Geometry: final body of the model. Coordinates: model frame, mm. Give positions to 0.01 mm unless a question says otherwise; leave off trailing zeros. Write each loop counter-clockwise with the first axis right and the second up, starting at its lowest first coordinate (ties: lowest second). Pieces come first, ordered by that corner, then holes. Notation, with made-up numbers: (-12, 84) -> (7, 84) arc R17 ccw to (7, 112) -> close; hole circle Ø3 at (52.5, 32). An arc over 180 degrees is marked (long way). Answer as a JSON object with one key per item and string values.
from build123d import *

# Parameters (mm, degrees)
BOSS_EXTRUDE1_DEPTH      = 2.159
BOSS_EXTRUDE1_DEPTH_BACK = 2.159
SKETCH6_W                = 177.8
SKETCH6_H                = 279.4
SKETCH6_W_2              = 152.4
SKETCH6_H_2              = 254
BOSS_EXTRUDE2_DEPTH      = 8.89
SKETCH7_R                = 3
CUT_EXTRUDE2_DEPTH       = 251.170207847


with BuildPart() as part:
    # Sketch3 → Boss-Extrude1 (new, two sides: drawn at the far end of the back side and taken through both)
    with BuildSketch(Plane.XY.offset(-BOSS_EXTRUDE1_DEPTH_BACK)):
        Polygon((-149.987, 177.025), (-126.987, 200.025), (126.987, 200.025), (149.987, 177.025), (149.987, -177.025), (126.987, -200.025), (-126.987, -200.025), (-149.987, -177.025), align=None)
    extrude(amount=BOSS_EXTRUDE1_DEPTH + BOSS_EXTRUDE1_DEPTH_BACK)

    # Sketch6 → Boss-Extrude2 (add)
    with BuildSketch(Plane(origin=(0, 0, -2.159), x_dir=(-1, 0, 0), z_dir=(0, 0, -1))):
        Rectangle(SKETCH6_W, SKETCH6_H)
        Rectangle(SKETCH6_W_2, SKETCH6_H_2, mode=Mode.SUBTRACT)
    extrude(amount=-BOSS_EXTRUDE2_DEPTH)

    # Sketch7 → Cut-Extrude2 (cut, through all)
    with BuildSketch(Plane(origin=(0, 0, -2.159), x_dir=(-1, 0, 0), z_dir=(0, 0, -1))):
        with Locations((133.477, 178.943)):
            Circle(SKETCH7_R)
        with Locations((-133.477, 178.943)):
            Circle(SKETCH7_R)
        with Locations((-133.477, -178.943)):
            Circle(SKETCH7_R)
        with Locations((133.477, -178.943)):
            Circle(SKETCH7_R)
    extrude(amount=-CUT_EXTRUDE2_DEPTH, mode=Mode.SUBTRACT)


solid = part.part
Q1. Cut plane B-B (y = -116). Return the cut outline in (x, z).
Values:
{"outline": "(-149.99, -2.16) -> (149.99, -2.16) -> (149.99, 2.16) -> (88.9, 2.16) -> (88.9, 6.73) -> (76.2, 6.73) -> (76.2, 2.16) -> (-76.2, 2.16) -> (-76.2, 6.73) -> (-88.9, 6.73) -> (-88.9, 2.16) -> (-149.99, 2.16) -> close"}
Q2. Cut plane D-D (x = -101.5). Return the cut outline in (y, z) (3 decimals).
Values:
{"outline": "(-200.025, -2.159) -> (200.025, -2.159) -> (200.025, 2.159) -> (-200.025, 2.159) -> close"}
Q3. First-contact query: P1, Ø5, axis at y = 61, z = 4.5, coming from the -X side; P2, Ø1.4, axis at x = 24, z = 5.5, coming from the -Y side; P3, Ø3.5, axis at y = -23.5, z = 5, coming from the -X side; P4, Ø8, axis at x = 133.477, y = 178.943, coming from the +Z side. Flat tips, straight axial feed; report the tip coordinate or a pass-through.
Values:
{"P1": "x = -149.99", "P2": "y = -139.7", "P3": "x = -88.9", "P4": "z = 2.16"}
Q4. Cut plane C-C (x = -66). Return the cut outline in (y, z) (3 decimals), and give its area (3 significant figures).
Values:
{"outline": "(-200.025, -2.159) -> (200.025, -2.159) -> (200.025, 2.159) -> (139.7, 2.159) -> (139.7, 6.731) -> (127, 6.731) -> (127, 2.159) -> (-127, 2.159) -> (-127, 6.731) -> (-139.7, 6.731) -> (-139.7, 2.159) -> (-200.025, 2.159) -> close", "area": "1,840 mm²"}
Q5. Cut plane A-A (z = 4). Return the cut outline in (x, y), and give its area (3 significant figures).
Values:
{"outline": "(-88.9, -139.7) -> (88.9, -139.7) -> (88.9, 139.7) -> (-88.9, 139.7) -> close; hole (-76.2, -127) -> (76.2, -127) -> (76.2, 127) -> (-76.2, 127) -> close", "area": "11,000 mm²"}
Q6. Mould query, pull axis X, two halves, no side actions, for faces 1 (the flat face through (79, 11, 6.731)), 2 (the flat face through (138.65, -188.36, -0.03)), 3 (the flat face through (1, 2, 2.159)). Classes: pulls with the +X half, pulls with the -X half, needs draft (parallel to the pull), parting line crosses it, or undercut.
Values:
{"face 1": "needs draft", "face 2": "pulls with the +X half", "face 3": "undercut"}
Q7. Material intervals for L1, parallel to X at y = -91.5, z = 5; L2, parallel to Y at x = 133, z = 1.25; L3, parallel to Y at x = -39.5, z = 3.75, sorted ascending. Write a range as from..to.
Values:
{"L1": "-88.9..-76.2, 76.2..88.9", "L2": "-194.01..-181.9, -175.98..175.98, 181.9..194.01", "L3": "-139.7..-127, 127..139.7"}
